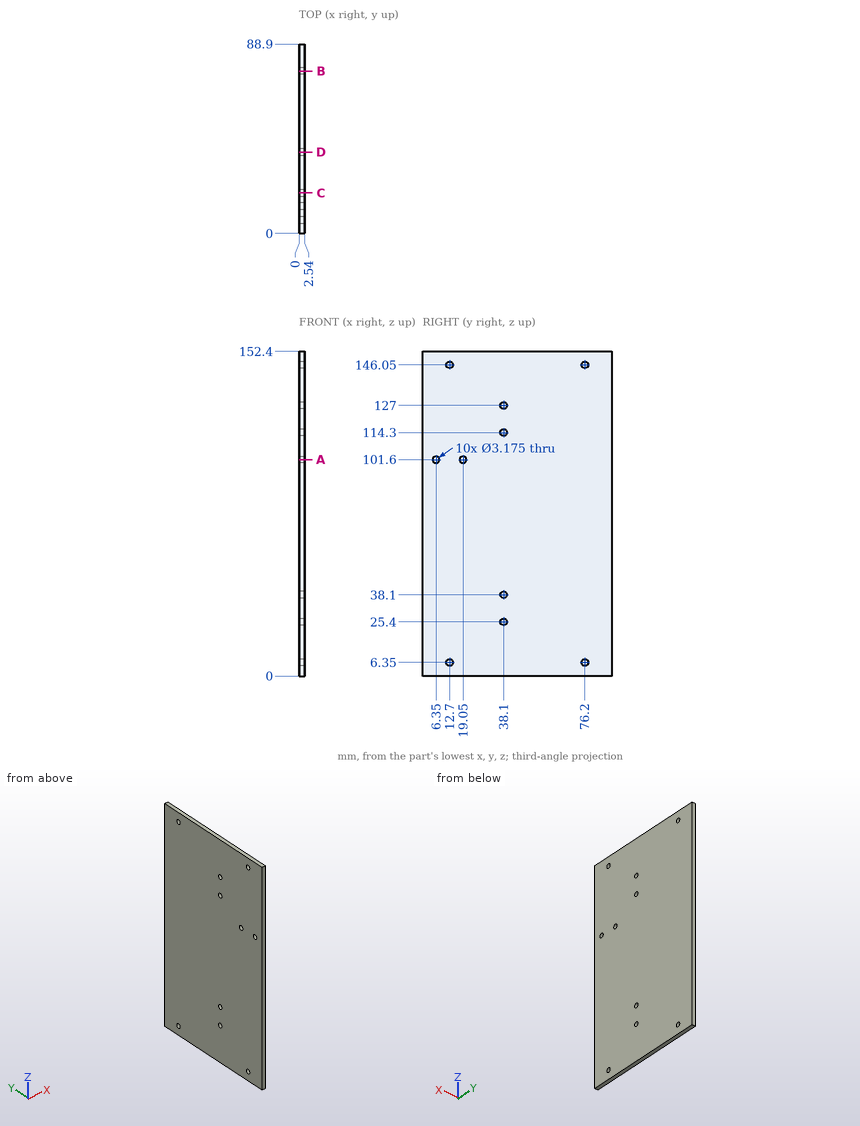
Verification items for this drawing (mm, ordinates from the low corner). Round coordinates to 2 decimals unless told otherwise and drop trailing zeros. Write each loop counter-clockwise with the first axis right and the second up, starting at its lowest first coordinate (ties: lowest second). Pieces come first, ordered by that corner, then holes. Notation, with made-up numbers: (-23.5, -8.75) - (11.5, -8.75) arc R8 ccw to (11.5, 6.25) - close; hole circle Ø11 at (68.5, 19.25). An arc over 180 degrees is marked (long way). Answer as a JSON object with one key per item and string values. Group by question number.
Q1. Go/stop test with flat-tipped pins: pin 1 Ø3 at (y, z) = (6.35, 101.6) entering from +X; pin 2 Ø4 at (y, z) = (19.05, 101.6) entering from +X. Record where each tip stops, or that it passes through.
Q2. Section check C-C, the plane y = 19.05. Enter the section's corners in (x, z).
Q3. Section check A-A, the plane z = 101.6. Enter the section's corners in (x, y).
Q4. Section check D-D, the plane y = 38.1. Enter the section's corners in (x, z), plus the area to 3 significant figures.
Q5. Section check B-B, the plane y = 76.2. Enter the section's corners in (x, z).
Q6. Thickness scan on line 1 (Y direction, x = 0.6, z = 6.35); line 2 (Z direction, x = 1.4, y = 76.2); line 3 (Y direction, x = 0.95, z = 38.1). Record the ranges inside material, lowest first.
Found:
{
 "1": {"pin 1": "passes through", "pin 2": "stops at x = 2.54"},
 "2": {"outline": "(0, 0) - (2.54, 0) - (2.54, 100.01) - (0, 100.01) - close; (0, 103.19) - (2.54, 103.19) - (2.54, 152.4) - (0, 152.4) - close"},
 "3": {"outline": "(0, 0) - (2.54, 0) - (2.54, 4.76) - (0, 4.76) - close; (0, 7.94) - (2.54, 7.94) - (2.54, 17.46) - (0, 17.46) - close; (0, 20.64) - (2.54, 20.64) - (2.54, 88.9) - (0, 88.9) - close"},
 "4": {"outline": "(0, 0) - (2.54, 0) - (2.54, 23.81) - (0, 23.81) - close; (0, 26.99) - (2.54, 26.99) - (2.54, 36.51) - (0, 36.51) - close; (0, 39.69) - (2.54, 39.69) - (2.54, 112.71) - (0, 112.71) - close; (0, 115.89) - (2.54, 115.89) - (2.54, 125.41) - (0, 125.41) - close; (0, 128.59) - (2.54, 128.59) - (2.54, 152.4) - (0, 152.4) - close", "area": "355 mm^2"},
 "5": {"outline": "(0, 0) - (2.54, 0) - (2.54, 4.76) - (0, 4.76) - close; (0, 7.94) - (2.54, 7.94) - (2.54, 144.46) - (0, 144.46) - close; (0, 147.64) - (2.54, 147.64) - (2.54, 152.4) - (0, 152.4) - close"},
 "6": {"line 1": "y = 0 to 11.11, 14.29 to 74.61, 77.79 to 88.9", "line 2": "z = 0 to 4.76, 7.94 to 144.46, 147.64 to 152.4", "line 3": "y = 0 to 36.51, 39.69 to 88.9"}
}
